Verification items for this drawing (mm, ordinates from the low corner). Coordinates: 2 decimals unless noted, no trailing zeros. Loops run counter-clockwise (first coordinate to the right, second up) from the corner with the lowest first, then second, coordinate; pieces in that order, holes last. Notation, with made-up numbers: M -18,60 L -3,60 A7 cw -3,65 Z; hole C 31,-32.75 d11. An arc over 180 degrees is marked long. Return JSON: item names as keys, results as strings.
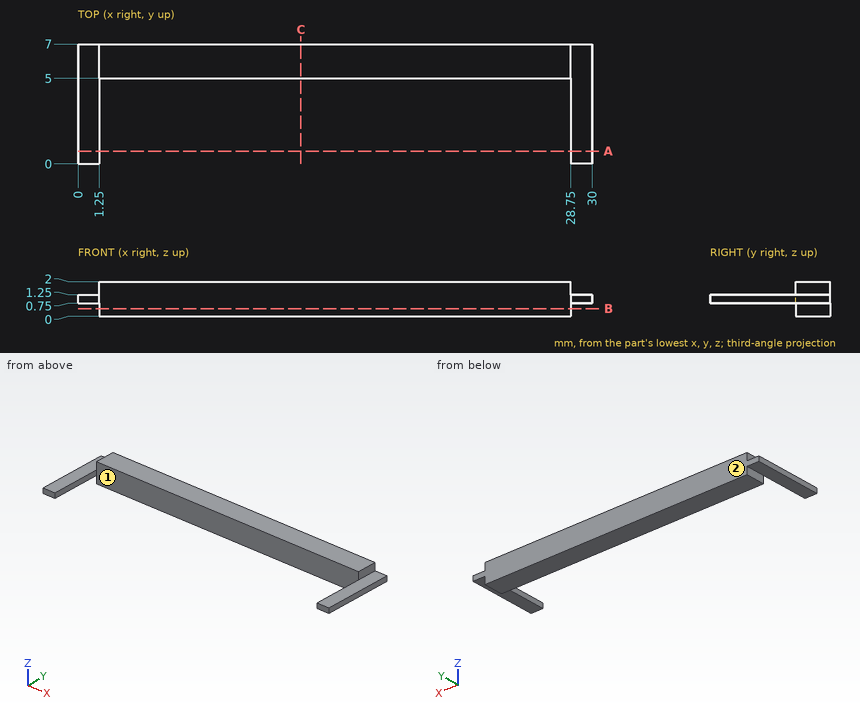
1) Scan lines: line 1 along X through (y, z) = (6.75, 1.85); line 2 along Y through (x, z) = (12.5, 0.6). Record each from-to range of solid material in increasing order. Write a range as [from, to].
Answers:
{"line 1": "[1.25, 28.75]", "line 2": "[5, 7]"}
2) Section check C-C on x = 13. Record the cut outline in (y, z), then the cut area to 3 significant figures.
Answers:
{"outline": "M 5,0 L 7,0 L 7,2 L 5,2 Z", "area": "4.00 mm²"}
3) Section check A-A on y = 0.75. Record the cut outline in (x, z), then the cut area to 3 significant figures.
Answers:
{"outline": "M 0,0.75 L 1.25,0.75 L 1.25,1.25 L 0,1.25 Z; M 28.75,0.75 L 30,0.75 L 30,1.25 L 28.75,1.25 Z", "area": "1.25 mm²"}
4) Section check B-B on z = 0.45. Record the cut outline in (x, y), then the cut area to 3 significant figures.
Answers:
{"outline": "M 1.25,5 L 28.75,5 L 28.75,7 L 1.25,7 Z", "area": "55.0 mm²"}
5) Draft check along X on the marked faces 1 and 2. Enter one of: +X half, -X half, draft (parallel to the pull), parting line (faces both ways), or undercut.
Answers:
{"face 1": "undercut", "face 2": "draft"}
6) Go/stop test with flat-tipped pins: pin 1 Ø1.4 at (x, y) = (0.5, 3) entering from +Z; pin 2 Ø1.4 at (x, y) = (29.5, 4) entering from -Z; pin 3 Ø0.6 at (x, z) = (18.5, 1.5) entering from -Y. Record where each tip stops, or that it passes through.
Answers:
{"pin 1": "z = 1.25", "pin 2": "z = 0.75", "pin 3": "y = 5"}
